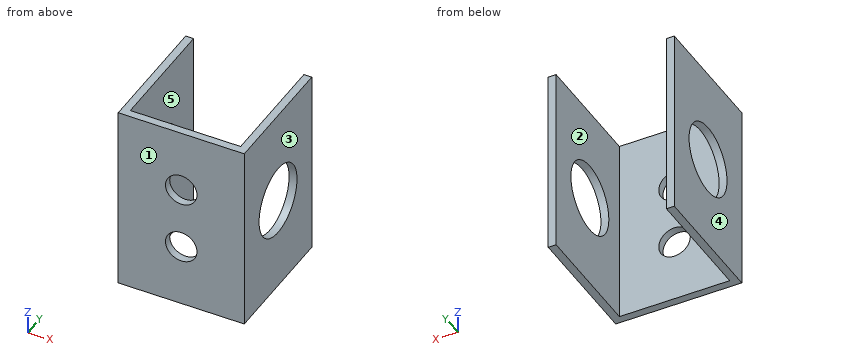
Autodesk Inventor part; units mm, degrees
ref_plane "YZ Plane" through (0, 0, 0) normal (1, 0, 0) x (0, 1, 0)
ref_plane "XZ Plane" through (0, 0, 0) normal (0, 1, 0) x (-1, 0, 0)
ref_plane "XY Plane" through (0, 0, 0) normal (0, 0, 1) x (1, 0, 0)
sketch "Sketch1" plane through (0, 0, 0) normal (0, 1, 0) x (-1, 0, 0)
  line L0 (0, 0) -> (50.8, 0)
  line L1 (50.8, 0) -> (50.8, -76.2)
  line L2 (50.8, -76.2) -> (0, -76.2)
  line L3 (0, -76.2) -> (0, 0)
  circle A0 centre (25.4, -50.8) radius 6.35
  circle A1 centre (25.4, -25.4) radius 6.35
  dimension "d0" = 50.8
  dimension "d1" = 76.2
  dimension "d13" = 25.4
  dimension "d14" = 25.4
  dimension "d15" = 25.4
  dimension "d16" = 25.4
  dimension "d17" = 12.7
  dimension "d18" = 12.7
extrude "Extrusion3" add sketch "Sketch1" along normal blind 3.175
sketch "Sketch5" plane through (0, 3.175, 0) normal (0, 1, 0) x (1, 0, 0)
  line L0 (0, 76.2) -> (-50.8, 76.2)
  line L1 (-50.8, 76.2) -> (-47.625, 76.2)
  line L2 (-47.625, 76.2) -> (-47.625, 0)
  line L3 (-47.625, 0) -> (-50.8, 0)
  line L4 (-50.8, 0) -> (-50.8, 76.2)
  line L5 (0, 76.2) -> (-3.175, 76.2)
  line L6 (-3.175, 76.2) -> (-3.175, 0)
  line L7 (-3.175, 0) -> (0, 0)
  line L8 (0, 0) -> (0, 76.2)
  point P0 (0, 0)
  dimension "d21" = 3.175
  dimension "d22" = 3.175
  dimension "d23" = 76.2
  dimension "d24" = 76.2
extrude "Extrusion4" add sketch "Sketch5" along normal blind 47.625
sketch "Sketch6" plane through (-50.8, 0, -76.2) normal (-1, 0, 0) x (0, 0, 1)
  circle A0 centre (38.1, 25.4) radius 14.2748
  line L0 (76.2, 0) -> (76.2, 50.8)
  line L1 (76.2, 0) -> (0, 0)
  dimension "d27" = 28.5496
  dimension "d28" = 38.1
  dimension "d29" = 25.4
extrude "Extrusion6" cut sketch "Sketch6" against normal blind 50.8
equation "\"d24\" = d23"
properties part number "Scaling Arms Mounting Bracket"
The model under review builds one solid part; all positions refer to its coordinate system, in mm. Face numbers are marked on the shaded views. A direction names the side the tool comes from. Coordinates: 2 decimals unless noted, no trailing zeros. Loops run counter-clockwise (first coordinate to the right, second up) from the corner with the lowest first, then second, coordinate; pieces in that order, holes last.
(1) Consider section B-B, the plane y = 25.4. Give the boundary of the cut face in (x, z) (3 decimals), plus the area to 3 significant figures.
Determined:
outline: (-50.8, -76.2) - (-47.625, -76.2) - (-47.625, -52.375) - (-50.8, -52.375) - close; (-50.8, -23.825) - (-47.625, -23.825) - (-47.625, 0) - (-50.8, 0) - close; (-3.175, -76.2) - (0, -76.2) - (0, -52.375) - (-3.175, -52.375) - close; (-3.175, -23.825) - (0, -23.825) - (0, 0) - (-3.175, 0) - close
area: 303 mm2
(2) Consider section C-C, the plane z = -38.1. Give the boundary of the cut face in (x, y) (3 decimals).
Determined:
outline: (-50.8, 0) - (0, 0) - (0, 11.125) - (-3.175, 11.125) - (-3.175, 3.175) - (-47.625, 3.175) - (-47.625, 11.125) - (-50.8, 11.125) - close; (-50.8, 39.675) - (-47.625, 39.675) - (-47.625, 50.8) - (-50.8, 50.8) - close; (-3.175, 39.675) - (0, 39.675) - (0, 50.8) - (-3.175, 50.8) - close
(3) Draft analysis for pull direction X (two halves, no side actions). For the marked faces 3, 4 and 5, state which applies: +X half, -X half, draft (parallel to the pull), parting line (faces both ways), or undercut.
Determined:
face 3: +X half
face 4: -X half
face 5: undercut
(4) Consider section D-D, the plane y = 9.5. Give the boundary of the cut face in (x, z) (3 decimals).
Determined:
outline: (-50.8, -76.2) - (-47.625, -76.2) - (-47.625, 0) - (-50.8, 0) - close; (-3.175, -76.2) - (0, -76.2) - (0, 0) - (-3.175, 0) - close
(5) Tool access review of the marked faces 1 and 2: name each direction out of +Z, -Z, +X, -X, +Y, -Y from which nothing blocks a thin tool from reaching the whole face with its end or side.
Determined:
face 1: +Z, -Z, +X, -X, -Y
face 2: +Z, -Z, +Y
(6) Consider section A-A, the plane x = -25.4. Give the boundary of the cut face in (y, z) (3 decimals).
Determined:
outline: (0, -76.2) - (3.175, -76.2) - (3.175, -57.15) - (0, -57.15) - close; (0, -44.45) - (3.175, -44.45) - (3.175, -31.75) - (0, -31.75) - close; (0, -19.05) - (3.175, -19.05) - (3.175, 0) - (0, 0) - close
(7) Wall thickness on L1, parallel to Z at x = -25, y = 1; L2, parallel to X at y = 11, z = -55 (3 decimals); L3, parallel to Y at x = -1.3, z = -38.1: over which ranges is each line inside the solid? List them lowest first.
Determined:
L1: z = -76.2 to -57.14, -44.46 to -31.74, -19.06 to 0
L2: x = -50.8 to -47.625, -3.175 to 0
L3: y = 0 to 11.13, 39.67 to 50.8
